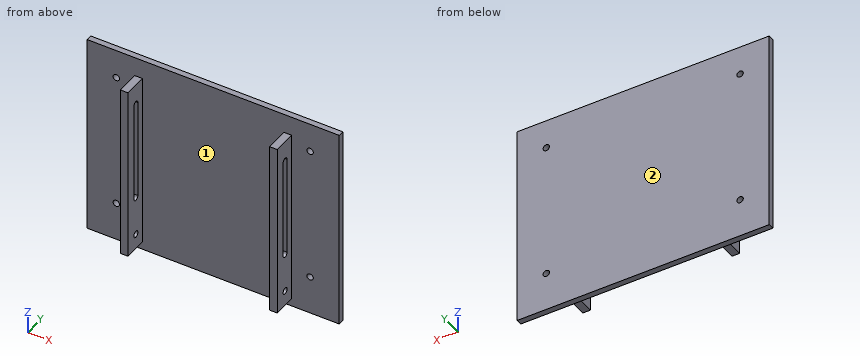
from build123d import *

# Parameters (mm, degrees)
SKETCH_1_W         = 130
SKETCH_1_H         = 105
F_3MM_DEPTH        = 3
SKETCH_2_W         = 4
SKETCH_2_H         = 91
F_12MM_DEPTH       = 12
SKETCH_3_R         = 1.65
F_3P3MM_DEPTH      = 142.149743181
SKETCH_4_R         = 1.65
CUT_EXTRUDE1_DEPTH = 115.450862819


with BuildPart() as part:
    # 草图1 → 支架连接板_3mm (new body)
    with BuildSketch(Plane(origin=(0, 0, 0), x_dir=(1, 0, 0), z_dir=(0, 1, 0))):
        with Locations((0, -40.5)):
            Rectangle(SKETCH_1_W, SKETCH_1_H)
    extrude(amount=F_3MM_DEPTH)

    # 草图2 → 左右导轨_12mm (add)
    with BuildSketch(Plane(origin=(0, 0, 0), x_dir=(1, 0, 0), z_dir=(0, 1, 0))):
        with Locations((-38.5, -37.5)):
            Rectangle(SKETCH_2_W, SKETCH_2_H)
        with Locations((38.5, -37.5)):
            Rectangle(SKETCH_2_W, SKETCH_2_H)
    extrude(amount=-F_12MM_DEPTH)

    # 草图3 → 左右铰接孔及滑槽_3p3mm (cut, through all)
    with BuildSketch(Plane(origin=(40.5, 0, 0), x_dir=(0, 0, -1), z_dir=(1, 0, 0))):
        with Locations((0, -5.5)):
            Circle(SKETCH_3_R)
        with BuildLine():
            Line((-20.48913575, -7.15), (-72.18913575, -7.15))
            ThreePointArc((-72.18913575, -7.15), (-73.83913575, -5.5), (-72.18913575, -3.85))
            Line((-72.18913575, -3.85), (-20.48913575, -3.85))
            ThreePointArc((-20.48913575, -3.85), (-18.83913575, -5.5), (-20.48913575, -7.15))
        make_face()
    extrude(amount=-F_3P3MM_DEPTH, mode=Mode.SUBTRACT)

    # 草图4 → Cut-Extrude1 (cut, through all)
    with BuildSketch(Plane(origin=(0, 3, 0), x_dir=(1, 0, 0), z_dir=(0, 1, 0))):
        with Locations(Location((-50, -8, 0), (0, 0, 270))):
            Circle(SKETCH_4_R)
        with Locations(Location((-50, -78, 0), (0, 0, 270))):
            Circle(SKETCH_4_R)
        with Locations(Location((50, -8, 0), (0, 0, 270))):
            Circle(SKETCH_4_R)
        with Locations(Location((50, -78, 0), (0, 0, 270))):
            Circle(SKETCH_4_R)
    extrude(amount=-CUT_EXTRUDE1_DEPTH, mode=Mode.SUBTRACT)


solid = part.part
Design review of the part built by this model. Coordinates are the model's own, in mm. Face numbers are marked on the shaded views. Round coordinates to 2 decimals unless told otherwise and drop trailing zeros. Loops run counter-clockwise (first coordinate to the right, second up) from the corner with the lowest first, then second, coordinate; pieces in that order, holes last. Notation, with made-up numbers: M 25,77 L 60,77 A16 ccw 60,101 Z; hole C 32.5,45.5 d9. An arc over 180 degrees is marked long. Answer as a JSON object with one key per item and string values.
Item 1: Wall thickness on L1, parallel to X at y = 0.65, z = 8; L2, parallel to Y at x = 37.8, z = 0; L3, parallel to X at y = -9, z = 52.5: over which ranges is each line inside the solid? List them lowest first. Write a range as from..to.
Answer sheet:
{"L1": "x = -65..-51.65, -48.35..48.35, 51.65..65", "L2": "y = -12..-7.15, -3.85..3", "L3": "x = -40.5..-36.5, 36.5..40.5"}
Item 2: We need section A-A on z = 48. Give the boundary of the cut face in (x, y).
Answer sheet:
{"outline": "M -65,0 L -40.5,0 L -40.5,-3.85 L -36.5,-3.85 L -36.5,0 L 36.5,0 L 36.5,-3.85 L 40.5,-3.85 L 40.5,0 L 65,0 L 65,3 L -65,3 Z; M -40.5,-12 L -36.5,-12 L -36.5,-7.15 L -40.5,-7.15 Z; M 36.5,-12 L 40.5,-12 L 40.5,-7.15 L 36.5,-7.15 Z"}
Item 3: We need section D-D on z = 11. Give the boundary of the cut face in (x, y), and give its area (3 significant figures).
Answer sheet:
{"outline": "M -65,0 L -40.5,0 L -40.5,-12 L -36.5,-12 L -36.5,0 L 36.5,0 L 36.5,-12 L 40.5,-12 L 40.5,0 L 65,0 L 65,3 L -65,3 Z", "area": "486 mm^2"}
Item 4: We need section B-B on y = -1.5. Give the boundary of the cut face in (x, z).
Answer sheet:
{"outline": "M -40.5,-8 L -36.5,-8 L -36.5,83 L -40.5,83 Z; M 36.5,-8 L 40.5,-8 L 40.5,83 L 36.5,83 Z"}
Item 5: We need section C-C on x = 50. Give the boundary of the cut face in (y, z).
Answer sheet:
{"outline": "M 0,-12 L 3,-12 L 3,6.35 L 0,6.35 Z; M 0,9.65 L 3,9.65 L 3,76.35 L 0,76.35 Z; M 0,79.65 L 3,79.65 L 3,93 L 0,93 Z"}
Item 6: The part is to be moulded in two halves that separate along X. For the marked faces 1 and 2, say which applies: pulls with the +X half, pulls with the -X half, needs draft (parallel to the pull), parting line crosses it, or undercut.
Answer sheet:
{"face 1": "undercut", "face 2": "needs draft"}
Item 7: Clearance check with flat-ended pins moving along their axes: P1, Ø2, axis at x = 39, y = -4.5, coming from the +Z side; P2, Ø8, axis at y = -2, z = 80, coming from the -X side; P3, Ø4, axis at x = 50, z = 78, coming from the -Y side; P4, Ø4, axis at y = -5.5, z = 0, coming from the -X side. State where each tip first meets the part, or that it passes through.
Answer sheet:
{"P1": "stops at z = 83", "P2": "stops at x = -65", "P3": "stops at y = 0", "P4": "stops at x = -40.5"}
